Geometry: see drawing. Coordinates: mm, zero at the bounding-box minimum. Coordinates: 2 decimals unless noted, no trailing zeros. Order: outer loops, then holes, each group sorted by start corner. A loop starts at its lowest first (then second) coordinate and runs counter-clockwise, first axis right, second up. Notation, with made-up numbers: (50.5, -2) -> (77.5, -2) arc R34 cw to (77.5, 36) -> close; hole circle Ø1 at (-24.5, 42). An arc over 180 degrees is marked (long way). Write each question's results on one line, items separated by ' | '. Start each with the question number.
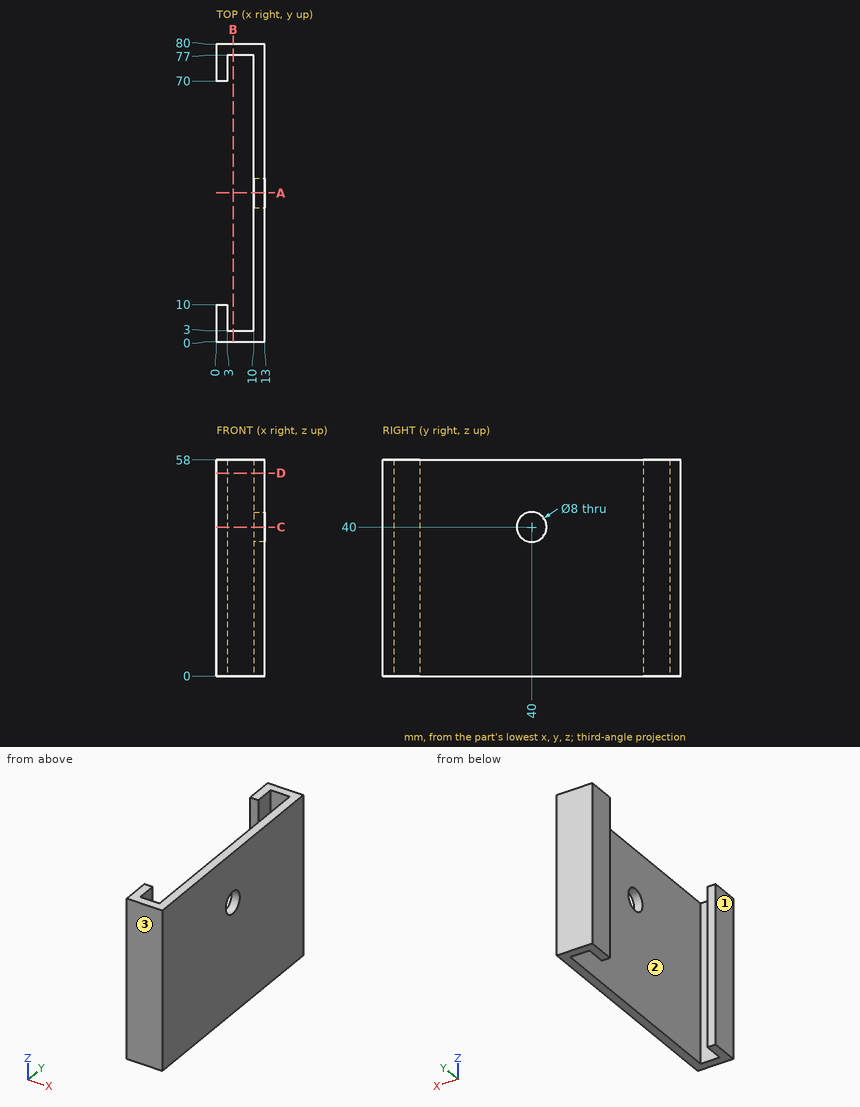
(1) Section D-D on z = 54.5. Return the cut outline in (x, y), then the cut area to 3 significant figures.
(2) Section B-B on x = 4.5. Return the cut outline in (y, z).
(3) Section C-C on z = 40. Return the cut outline in (x, y), then the cut area to 3 significant figures.
(4) Draft query along Y for the marked faces 1, 2 and 3. Return one class per face: released by +Y, released by -Y, zero draft, split by the parting line, or undercut.
(5) Section A-A on y = 40. Return the cut outline in (x, z), then the cut area to 3 significant figures.
(6) First-contact query: P1, Ø4, axis at x = 9.5, y = 48.5, coming from the -Z side; P2, Ø10, axis at y = 61.5, z = 41.5, coming from the -X side. Flat tips, straight axial feed; report the tip coordinate or a pass-through.
(7) Line query: L1, parallel to X at y = 71.5, z = 16; L2, parallel to Y at x = 10.95, z = 40; L3, parallel to Y at x = 0.5, z = 53. Output: solid intervals per line, ascending.
Results list:
1) outline: (0, 0) -> (13, 0) -> (13, 80) -> (0, 80) -> (0, 70) -> (3, 70) -> (3, 77) -> (10, 77) -> (10, 3) -> (3, 3) -> (3, 10) -> (0, 10) -> close | area: 342 mm²
2) outline: (0, 0) -> (3, 0) -> (3, 58) -> (0, 58) -> close; (77, 0) -> (80, 0) -> (80, 58) -> (77, 58) -> close
3) outline: (0, 0) -> (13, 0) -> (13, 36) -> (10, 36) -> (10, 3) -> (3, 3) -> (3, 10) -> (0, 10) -> close; (0, 70) -> (3, 70) -> (3, 77) -> (10, 77) -> (10, 44) -> (13, 44) -> (13, 80) -> (0, 80) -> close | area: 318 mm²
4) face 1: zero draft | face 2: undercut | face 3: released by -Y
5) outline: (10, 0) -> (13, 0) -> (13, 36) -> (10, 36) -> close; (10, 44) -> (13, 44) -> (13, 58) -> (10, 58) -> close | area: 150 mm²
6) P1: stops at z = 0 | P2: stops at x = 10
7) L1: x = 0 to 3, 10 to 13 | L2: y = 0 to 36, 44 to 80 | L3: y = 0 to 10, 70 to 80
